The model under review builds one solid part; all positions refer to its coordinate system, in mm. Face numbers are marked on the shaded views. A direction names the side the tool comes from. Coordinates: 2 decimals unless noted, no trailing zeros. Loops run counter-clockwise (first coordinate to the right, second up) from the corner with the lowest first, then second, coordinate; pieces in that order, holes last. Notation, with made-up numbers: (-11.5, -16) - (27.5, -16) arc R31 ccw to (27.5, 23) - close; hole circle Ø2 at (76.5, -22.5). An arc over 180 degrees is marked (long way). Answer in a Markdown table with one row per item. Add a question column.
(1) We need section B-B on x = 40. Write out the cut boundary in (y, z), plus the area to 3 significant figures.
(2) Machinability: for the marked faces 1 and 2, which of the approach directions +Z, -Z, +X, -X, +Y, -Y give a long, thin tool a straight path to every point of the face, cutting with its end or side? Answer none if there is none.
(3) For line 1 along Y through (x, z) = (40, -0.8); line 2 along Z through (x, y) = (32.5, 4.5); line 3 along X through (y, z) = (11.5, 18.25), list the stretches that pass through material, from the lowest coordinate up.
(4) We need section D-D on y = 25. Write out the cut boundary in (x, z), plus the area to 3 significant figures.
(5) We need section A-A on y = 15. Write out the cut boundary in (x, z).
(6) For P1, Ø1, axis at x = 34.5, y = 16.5, coming from the +Z side; P2, Ø3.5, axis at y = 5, z = 9.57, coming from the +X side, all flat-tipped, find the tip position at first contact; note any pin that passes through.
(7) We need section C-C on z = 10. Write out the cut boundary in (x, y), plus the area to 3 significant figures.
from build123d import *

# Parameters (mm, degrees)
BASE_FLANGE1_DEPTH              = 1.5
SKETCHED_BEND1_DEPTH            = 30
SKETCHED_BEND1_2_DEPTH          = 30
F_5_0MM_PRESS_DOWEL_HOLE1_D     = 5
F_3_0MM_PRESS_DOWEL_HOLE1_D     = 3
F_3_0MM_PRESS_DOWEL_HOLE2_D     = 3
F_3_0MM_PRESS_DOWEL_HOLE3_D     = 3
F_3_0MM_PRESS_DOWEL_HOLE3_DEPTH = 6
F_3_0MM_PRESS_DOWEL_HOLE3_TIP   = 0.901290929


# Read off the part's stored shape, not the designer's step: Sketched Bend1
# Sheet-metal steps are written as plain solids
with BuildPart() as part:
    # Sketch1 → Base-Flange1 (new body)
    with BuildSketch(Plane.XY):
        Polygon((0, 0), (25, 0), (55, 0), (55, 30), (25, 30), (0, 30), align=None)
    extrude(amount=-BASE_FLANGE1_DEPTH)

    # Sketched Bend1 outline → Sketched Bend1 (cut)
    with BuildSketch(Plane(origin=(0, 0, 0), x_dir=(1, 0, 0), z_dir=(0, 1, 0))):
        with BuildLine():
            Line((0, 0), (24.055749054, 0))
            ThreePointArc((24.055749054, 0), (24.872408828, 1.086838938), (26.16757291, 1.5))
            Line((26.16757291, 1.5), (0, 1.5))
            Line((0, 1.5), (0, 0))
        make_face()
    extrude(amount=SKETCHED_BEND1_DEPTH, mode=Mode.SUBTRACT)

    # Sketched Bend1 2 outline → Sketched Bend1 2 (add)
    with BuildSketch(Plane(origin=(0, 0, 0), x_dir=(1, 0, 0), z_dir=(0, 1, 0))):
        with BuildLine():
            ThreePointArc((24.055749054, 0), (23.962387567, -0.363053267), (23.93097291, -0.7366))
            Line((23.93097291, -0.7366), (23.93097291, -24.56902709))
            Line((23.93097291, -24.56902709), (25.43097291, -24.56902709))
            Line((25.43097291, -24.56902709), (25.43097291, -0.7366))
            ThreePointArc((25.43097291, -0.7366), (25.646718055, -0.215745145), (26.16757291, 0))
            Line((26.16757291, 0), (24.055749054, 0))
        make_face()
    extrude(amount=SKETCHED_BEND1_2_DEPTH)

    # Ø5.0mm Press Dowel Hole1 (through all)
    with Locations(Plane(origin=(0, 0, -1.5), x_dir=(-1, 0, 0), z_dir=(0, 0, -1))):
        with Locations((-39.93097291, 15)):
            Hole(F_5_0MM_PRESS_DOWEL_HOLE1_D / 2)

    # Ø3.0mm Press Dowel Hole1 (through all)
    with Locations(Plane(origin=(0, 0, -1.5), x_dir=(-1, 0, 0), z_dir=(0, 0, -1))):
        with Locations((-40, 4), (-40, 26)):
            Hole(F_3_0MM_PRESS_DOWEL_HOLE1_D / 2)

    # Ø3.0mm Press Dowel Hole2 (through all)
    with Locations(Plane(origin=(25.43097291, 0, 0), x_dir=(0, 0, -1), z_dir=(1, 0, 0))):
        with Locations((-9.56902709, 5), (-9.56902709, 25)):
            Hole(F_3_0MM_PRESS_DOWEL_HOLE2_D / 2)

    # Ø3.0mm Press Dowel Hole3
    with Locations(Plane(origin=(23.93097291, -205.525513363, -308.224624397), x_dir=(0, 1, 0), z_dir=(1, 0, 0))):
        with Locations((220.525513363, 156.531359221), (102.525513363, 181.531359221), (102.525513363, 271.531359221), (89.19270005, 226.531359221), (210.525513363, 317.793651488), (230.525513363, 317.793651488), (252.525513363, 320.462332131), (232.525513363, 300.462332131), (252.525513363, 132.600386311), (232.525513363, 152.600386311), (111.286271896, 136.531359221), (91.286271896, 136.531359221), (41.525513363, 196.432813402), (13.525513363, 196.432813402), (41.525513363, 138.767959221), (13.525513363, 138.767959221), (41.525513363, 256.62990504), (13.525513363, 256.62990504), (41.525513363, 314.294759221), (13.525513363, 314.294759221)):
            Hole(F_3_0MM_PRESS_DOWEL_HOLE3_D / 2, depth=F_3_0MM_PRESS_DOWEL_HOLE3_DEPTH)
            with Locations((0, 0, -(F_3_0MM_PRESS_DOWEL_HOLE3_DEPTH + F_3_0MM_PRESS_DOWEL_HOLE3_TIP / 2))):  # 118° drill point
                Cone(0, F_3_0MM_PRESS_DOWEL_HOLE3_D / 2, F_3_0MM_PRESS_DOWEL_HOLE3_TIP, mode=Mode.SUBTRACT)


solid = part.part
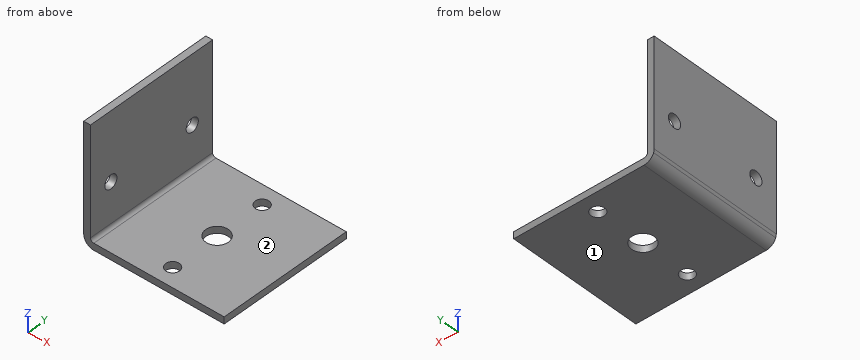
Outcome:
| question | item | result |
|---|---|---|
| 1 | outline | (0, -1.5) - (2.5, -1.5) - (2.5, 0) - (0, 0) - close; (5.5, -1.5) - (12.5, -1.5) - (12.5, 0) - (5.5, 0) - close; (17.5, -1.5) - (24.5, -1.5) - (24.5, 0) - (17.5, 0) - close; (27.5, -1.5) - (30, -1.5) - (30, 0) - (27.5, 0) - close |
| 1 | area | 28.5 mm² |
| 2 | face 1 | -Z, +X, -X, +Y, -Y |
| 2 | face 2 | +Z, +X, +Y, -Y |
| 3 | line 1 | 0 to 2.5, 5.5 to 12.5, 17.5 to 24.5, 27.5 to 30 |
| 3 | line 2 | -1.5 to 0 |
| 3 | line 3 | 23.93 to 25.43 |
| 4 | outline | (23.93, 0.74) arc R2.24 ccw to (26.17, -1.5) - (38.88, -1.5) - (38.88, 0) - (26.17, 0) arc R0.74 cw to (25.43, 0.74) - (25.43, 8.07) - (23.93, 8.07) - close; (23.93, 11.07) - (25.43, 11.07) - (25.43, 24.57) - (23.93, 24.57) - close; (41.12, -1.5) - (55, -1.5) - (55, 0) - (41.12, 0) - close |
| 4 | area | 74.6 mm² |
| 5 | outline | (23.93, 0.74) arc R2.24 ccw to (26.17, -1.5) - (37.43, -1.5) - (37.43, 0) - (26.17, 0) arc R0.74 cw to (25.43, 0.74) - (25.43, 24.57) - (23.93, 24.57) - close; (42.43, -1.5) - (55, -1.5) - (55, 0) - (42.43, 0) - close |
| 6 | P1 | z = 0 |
| 6 | P2 | x = 25.43 |
| 7 | outline | (23.93, 0) - (25.43, 0) - (25.43, 3.56) - (23.93, 3.56) - close; (23.93, 6.44) - (25.43, 6.44) - (25.43, 23.56) - (23.93, 23.56) - close; (23.93, 26.44) - (25.43, 26.44) - (25.43, 30) - (23.93, 30) - close |
| 7 | area | 36.4 mm² |
